Work out the finished part from the listing and answer in its coordinate system (mm). A direction names the side the tool comes from. Round coordinates to 2 decimals unless told otherwise and drop trailing zeros. Write each loop counter-clockwise with the first axis right and the second up, starting at its lowest first coordinate (ties: lowest second). Pieces come first, ordered by that corner, then holes. Notation, with made-up numbers: (48, 0) - (107, 0) arc R32 cw to (107, 26) - close; hole circle Ø6 at (70.25, 34.5). An arc over 180 degrees is marked (long way). Answer as a JSON object with one key per item and string values.
```python
from build123d import *

# Parameters (mm, degrees)
SKETCH1_W           = 80
SKETCH1_H           = 36
SKETCH1_R           = 1.5
SKETCH1_W_2         = 71
SKETCH1_H_2         = 24
BOSS_EXTRUDE1_DEPTH = 10
SKETCH1_3_W         = 71
SKETCH1_3_H         = 24
BOSS_EXTRUDE2_DEPTH = 7
BOSS_EXTRUDE3_DEPTH = 3


with BuildPart() as part:
    # Sketch1 → Boss-Extrude1 (new body)
    # profile 1 of 2: a face of its own
    with BuildSketch(Plane(origin=(0, 0, 0), x_dir=(1, 0, 0), z_dir=(0, 1, 0))):
        Rectangle(SKETCH1_W, SKETCH1_H)
        with Locations(Location((-37.5, 15.5, 0), (0, 0, 270))):
            Circle(SKETCH1_R, mode=Mode.SUBTRACT)
        with Locations(Location((-37.5, -15.5, 0), (0, 0, 270))):
            Circle(SKETCH1_R, mode=Mode.SUBTRACT)
        with Locations(Location((37.5, -15.5, 0), (0, 0, 270))):
            Circle(SKETCH1_R, mode=Mode.SUBTRACT)
        with Locations(Location((37.5, 15.5, 0), (0, 0, 270))):
            Circle(SKETCH1_R, mode=Mode.SUBTRACT)
        Rectangle(SKETCH1_W_2, SKETCH1_H_2, mode=Mode.SUBTRACT)
    # profile 2 of 2: a face of its own
    with BuildSketch(Plane(origin=(0, 0, 0), x_dir=(1, 0, 0), z_dir=(0, 1, 0))):
        Rectangle(SKETCH1_W_2, SKETCH1_H_2)
    extrude(amount=-BOSS_EXTRUDE1_DEPTH)

    # Sketch1_3 → Boss-Extrude2 (add)
    with BuildSketch(Plane(origin=(0, 0, 0), x_dir=(1, 0, 0), z_dir=(0, 1, 0))):
        Rectangle(SKETCH1_3_W, SKETCH1_3_H)
    extrude(amount=BOSS_EXTRUDE2_DEPTH)

    # Sketch2 → Boss-Extrude3 (add)
    with BuildSketch(Plane(origin=(0, 0, 0), x_dir=(1, 0, 0), z_dir=(0, 1, 0))):
        Polygon((-38.5, -1.5), (-35.5, -4), (-35.5, 0), (-38.5, 0), align=None)
        Polygon((-38.5, 0), (-35.5, 0), (-35.5, 4), (-38.5, 1.5), align=None)
    extrude(amount=BOSS_EXTRUDE3_DEPTH)


solid = part.part
```
Item 1: A cutting plane is placed at C-C (z = 8). Write down the section's boundary in (x, y).
Results found:
{"outline": "(-40, -10) - (40, -10) - (40, 0) - (35.5, 0) - (35.5, 7) - (-35.5, 7) - (-35.5, 0) - (-40, 0) - close"}
Item 2: A cutting plane is placed at A-A (z = 15.5). Write down the section's boundary in (x, y), and give its area (3 significant figures).
Results found:
{"outline": "(-40, -10) - (-39, -10) - (-39, 0) - (-40, 0) - close; (-36, -10) - (36, -10) - (36, 0) - (-36, 0) - close; (39, -10) - (40, -10) - (40, 0) - (39, 0) - close", "area": "740 mm²"}
Item 3: Each of these flat-tipped pins is pushed along its axis until it touches: P1, Ø3.5, axis at y = 2.5, z = 2, coming from the +X side; P2, Ø5, axis at x = -37.5, z = 15.5, coming from the -Y side; P3, Ø1.8, axis at x = 37.5, z = -15.5, coming from the -Y side; P4, Ø2, axis at x = 11.5, y = 4, coming from the -Z side. Where does it stop, or does it pass through?
Results found:
{"P1": "x = 35.5", "P2": "y = -10", "P3": "through", "P4": "z = -12"}
Item 4: A cutting plane is placed at D-D (x = -20). Write down the section's boundary in (y, z), and give its area (3 significant figures).
Results found:
{"outline": "(-10, -18) - (0, -18) - (0, -12) - (7, -12) - (7, 12) - (0, 12) - (0, 18) - (-10, 18) - close", "area": "528 mm²"}
Item 5: A cutting plane is placed at B-B (x = 37.5). Write down the section's boundary in (y, z).
Results found:
{"outline": "(-10, -18) - (0, -18) - (0, -17) - (-10, -17) - close; (-10, -14) - (0, -14) - (0, 14) - (-10, 14) - close; (-10, 17) - (0, 17) - (0, 18) - (-10, 18) - close"}
Item 6: Determine the mould class of faces 1 (the flat face through (-1, -5, -18)), 2 (the cylindrical face through (36.6, -4.9, -16.7)), 3 (the flat face through (-9.4, 0, -12.3)) for opening direction Z: pulls with the +Z half, pulls with the -Z half, needs draft (parallel to the pull), parting line crosses it, or undercut.
Results found:
{"face 1": "pulls with the -Z half", "face 2": "undercut", "face 3": "needs draft"}
Item 7: Consider line 1 along X through (y, z) = (-2.75, -15.5); line 2 along Z through (x, y) = (-26, 4.5); line 3 along X through (y, z) = (1.25, 11). Determine where each line is inside the solid, lowest interval first.
Results found:
{"line 1": "-40 to -39, -36 to 36, 39 to 40", "line 2": "-12 to 12", "line 3": "-35.5 to 35.5"}
Item 8: For faces 4 (the flat face through (35.5, 3, 0)), 5 (the flat face through (-37.021, 1.479, 2.732)), 6 (the flat face through (-37, 3, 0)), 7 (the flat face through (-36.979, 1.479, -2.768)), 8 (the flat face through (0, 3, -12)), determine the directions among +Z, -Z, +X, -X, +Y, -Y from which every point of the face is accessible in a straight line to the end or side of a thin tool.
Results found:
{"face 4": "+Z, -Z, +X, +Y", "face 5": "+Z, -X, +Y", "face 6": "+Z, -Z, -X, +Y", "face 7": "-Z, -X, +Y", "face 8": "-Z, +X, -X, +Y"}
